Geometry: final body of the model. Coordinates: model frame, mm. A direction names the side the tool comes from. Give positions to 0.01 mm unless a question says otherwise; leave off trailing zeros. Loops run counter-clockwise (first coordinate to the right, second up) from the corner with the lowest first, then second, coordinate; pieces in that order, holes last.
1. First-contact query: P1, Ø16, axis at x = 4, y = 30.5, coming from the -Z side; P2, Ø1.9, axis at x = -3, z = 108, coming from the -Y side; P3, Ø5, axis at x = -7.75, z = 116, coming from the +Y side. Flat tips, straight axial feed; report the tip coordinate or a pass-through.
2. Material intervals for line 1 along Y through (x, z) = (-1, 118); line 2 along X through (y, z) = (-23, 100); line 3 along X through (y, z) = (23, 93), sorted ascending.
3. Access query for faces 3 (the face through (11, 28, 126)), 4 (the face through (11.131, -55.528, 114.997)), 5 (the face through (0.808, -23.965, 90.978)), 6 (the face through (13, 0, 108)), 7 (the face through (15, 35, 108)). Directions: +Z, -Z, +X, -X, +Y, -Y. A direction counts if a zero-diameter tool reaches every point of the face in a straight line with its end or side. Return the directions, or none.
4. Section C-C, the plane y = -47. Output: boundary loops of the cut face in (x, z), then the cut area to 3 significant figures.
5. Draft query along Z for faces 1 (the face through (7.845, -23.528, 94.124)), 2 (the face through (-12, -55, 108)). Return one class per face: +Z half, -Z half, draft (parallel to the pull), parting line (faces both ways), or undercut.
6. Section B-B, the plane z = 108. State how many separate pieces and enclosed holes the cut face has, then the cut area to 3 significant figures.
7. Section A-A, the plane y = -31.5. Output: boundary loops of the cut face in (x, z).
from build123d import *

# Parameters (mm, degrees)
SKETCH_W               = 51
SKETCH_H               = 40
PAD_DEPTH              = 6
SKETCH002_W            = 4
SKETCH002_H            = 40
PAD001_DEPTH           = 25
PAD009_DEPTH           = 20
SKETCH031_W            = 5.9
SKETCH031_H            = 12.9
POCKET009_DEPTH        = 40
PAD010_DEPTH           = 12
SKETCH032_R            = 1.6
SKETCH032_R_2          = 1.025
POCKET010_DEPTH        = 5
SKETCH033_R            = 1.6
POCKET011_DEPTH        = 5
POCKET012_DEPTH        = 5
SKETCH042_R            = 1.6
POCKET019_DEPTH        = 5
SKETCH043_R            = 1.025
POCKET020_DEPTH        = 5
LINEARPATTERN004_COUNT = 2
LINEARPATTERN004_PITCH = 32
SKETCH044_W            = 4
SKETCH044_H            = 32
PAD015_DEPTH           = 27
SKETCH045_R            = 6
SKETCH045_R_2          = 2.1
POCKET021_DEPTH        = 5
FILLET001_R            = 1


with BuildPart() as part:
    # Sketch → Pad (new body)
    with BuildSketch(Plane.YZ):
        Rectangle(SKETCH_W, SKETCH_H)
    extrude(amount=PAD_DEPTH)

    # Sketch002 (on Face5 of Pad) → Pad001 (join)
    with BuildSketch(Plane(origin=(0, 0, 0), x_dir=(0, 1, 0), z_dir=(-1, 0, 0))):
        with Locations((23.5, 0)):
            Rectangle(SKETCH002_W, SKETCH002_H)
        with Locations((-23.5, 0)):
            Rectangle(SKETCH002_W, SKETCH002_H)
    extrude(amount=PAD001_DEPTH)

    # Sketch030 (on Face9 of Pad001) → Pad009 (join)
    with BuildSketch(Plane.ZX.offset(25.5)):
        Polygon((-16, -25), (-20, -25), (-20, 6), (20, 6), (20, -25), (16, -25), (16, 2), (-16, 2), align=None)
    pad009 = extrude(amount=PAD009_DEPTH)

    # Sketch031 (on Face12 of Pad009) → Pocket009 (cut)
    with BuildSketch(Plane.YX.offset(20)):
        Polygon((27.5, -25), (45.5, 0), (45.5, -25), align=None)
        with Locations((28.45, -8.45)):
            Rectangle(SKETCH031_W, SKETCH031_H)
    extrude(amount=-POCKET009_DEPTH, mode=Mode.SUBTRACT)

    # Mirrored: Pad009 across XZ
    add(pad009.mirror(Plane.XZ))

    # Mirrored Face21 → Pad010 (add)
    with BuildSketch(Plane(origin=(-4.904255, -45.5, 0), x_dir=(-1, 0, 0), z_dir=(0, -1, 0))):
        Polygon((20.095745, 16), (20.095745, 20), (-10.904255, 20), (-10.904255, -20), (20.095745, -20), (20.095745, -16), (-6.904255, -16), (-6.904255, 16), align=None)
    extrude(amount=PAD010_DEPTH)

    # Sketch032 (on Face19 of Pad010) → Pocket010 (cut)
    with BuildSketch(Plane(origin=(0, -25.5, 0), x_dir=(0, 0, -1), z_dir=(0, -1, 0))):
        with Locations((-8, -5.75)):
            Circle(SKETCH032_R)
        with Locations((8, -5.75)):
            Circle(SKETCH032_R)
        with Locations((8, -20.75)):
            Circle(SKETCH032_R)
        with Locations((-8, -20.75)):
            Circle(SKETCH032_R)
        with Locations((-14.9, -5.2)):
            Circle(SKETCH032_R_2)
        with Locations((-14.9, -11.7)):
            Circle(SKETCH032_R_2)
        with Locations((14.9, -5.2)):
            Circle(SKETCH032_R_2)
        with Locations((14.9, -11.7)):
            Circle(SKETCH032_R_2)
        with Locations((0, -16)):
            Circle(SKETCH032_R)
        with Locations((0, -22)):
            Circle(SKETCH032_R)
    pocket010 = extrude(amount=-POCKET010_DEPTH, mode=Mode.SUBTRACT)

    # Mirrored001: Pocket010 across XZ
    add(pocket010.mirror(Plane.XZ), mode=Mode.SUBTRACT)

    # Sketch033 (on Face30 of Mirrored001) → Pocket011 (cut)
    with BuildSketch(Plane.YZ.offset(6)):
        with Locations((-27, 8.5)):
            Circle(SKETCH033_R)
        with Locations((28, 8.5)):
            Circle(SKETCH033_R)
        with Locations((28, -8.5)):
            Circle(SKETCH033_R)
        with Locations((-27, -8.5)):
            Circle(SKETCH033_R)
    extrude(amount=-POCKET011_DEPTH, mode=Mode.SUBTRACT)

    # Sketch034 (on Face48 of Pocket011) → Pocket012 (cut)
    with BuildSketch(Plane(origin=(2, 0, 0), x_dir=(0, 1, 0), z_dir=(-1, 0, 0))):
        Polygon((-27.5, -5.42), (-30.167358, -6.96), (-30.167358, -10.04), (-27.5, -11.58), (-24.832642, -10.04), (-24.832642, -6.96), align=None)
    extrude(amount=POCKET012_DEPTH, mode=Mode.SUBTRACT)

    # Sketch042 (on Face13 of Pocket012) → Pocket019 (cut)
    with BuildSketch(Plane.YX.offset(20)):
        with Locations((-31.5, -12.5)):
            Circle(SKETCH042_R)
        with Locations((-51.5, -12.5)):
            Circle(SKETCH042_R)
    pocket019 = extrude(amount=-POCKET019_DEPTH, mode=Mode.SUBTRACT)

    # Mirrored005: Pocket019 across XY
    add(pocket019.mirror(Plane.XY), mode=Mode.SUBTRACT)

    # Sketch043 (on Face27 of Mirrored005) → Pocket020 (cut)
    with BuildSketch(Plane.ZX.offset(-21.5)):
        with Locations((-18, -12.5)):
            Circle(SKETCH043_R)
        with Locations((-18, -4.5)):
            Circle(SKETCH043_R)
    pocket020 = extrude(amount=-POCKET020_DEPTH, mode=Mode.SUBTRACT)

    # LinearPattern004: Pocket020 ×2
    with Locations(*[(0, -i * LINEARPATTERN004_PITCH, 0) for i in range(1, LINEARPATTERN004_COUNT)]):
        add(pocket020, mode=Mode.SUBTRACT)

    # Sketch044 (on Face54 of LinearPattern004) → Pad015 (join)
    with BuildSketch(Plane(origin=(2, 0, 0), x_dir=(0, 1, 0), z_dir=(-1, 0, 0))):
        with Locations((-55.5, 0)):
            Rectangle(SKETCH044_W, SKETCH044_H)
    extrude(amount=PAD015_DEPTH)

    # Sketch045 (on Face64 of Pad015) → Pocket021 (cut)
    with BuildSketch(Plane(origin=(0, -57.5, 0), x_dir=(0, 0, -1), z_dir=(0, -1, 0))):
        with Locations((0, -11.5)):
            Circle(SKETCH045_R)
        with Locations((-9, -2.5)):
            Circle(SKETCH045_R_2)
        with Locations((9, -2.5)):
            Circle(SKETCH045_R_2)
        with Locations((9, -20.5)):
            Circle(SKETCH045_R_2)
        with Locations((-9, -20.5)):
            Circle(SKETCH045_R_2)
    extrude(amount=-POCKET021_DEPTH, mode=Mode.SUBTRACT)

    # Fillet001
    fillet001_edges = [part.edges().sort_by_distance(p)[0] for p in [
        (-25, -57.5, 0),
        (6, -6, -20),
        (-9.5, -57.5, 20),
        (6, -6, 20),
        (-25, -39.5, 20),
        (-25, -39.5, -20),
        (-25, -21.5, 0),
        (-25, 27.5, -18),
        (-12.5, 36.5, -20),
        (-25, 25.5, 0),
        (-25, 27.5, 18),
        (3, 45.5, -20),
        (3, 45.5, 20),
        (-12.5, 36.5, 20),
        (0, 0, 20),
        (0, 0, -20),
        (6, -57.5, 0),
        (-25, 24.5, 20),
        (-25, 24.5, -20),
        (-25, 21.5, 0),
        (2, 45.5, 0),
        (-12.5, 36.5, 16),
        (-12.5, 36.5, -16),
        (0, 45.5, -18),
        (0, 45.5, 18),
        (1, 45.5, 16),
        (6, 45.5, 0),
    ]]
    fillet(fillet001_edges, radius=FILLET001_R)


with BuildPart() as part_1:
    # Body placement: moved
    add(part.part.moved(Location((13, 0, 108))))


solid = part_1.part
Answers below:
1. P1: stops at z = 88
1. P2: passes through
1. P3: stops at y = 25.5
2. line 1: y = -57.5 to -53.5, -25.5 to -21.5, 21.5 to 25.5
2. line 2: x = -12 to -9.35, -6.15 to 5.65, 8.85 to 19
2. line 3: x = -12 to 0.28, 2.32 to 6.78, 8.82 to 19
3. face 3: +Z, -Z
3. face 4: -Y
3. face 5: none
3. face 6: +Z, -Z, -X
3. face 7: -X, +Y
4. outline: (-12, 89) arc R1 ccw to (-11, 88) - (18, 88) arc R1 ccw to (19, 89) - (19, 127) arc R1 ccw to (18, 128) - (-11, 128) arc R1 ccw to (-12, 127) - (-12, 124) - (15, 124) - (15, 92) - (-12, 92) - close
4. area: 375 mm2
5. face 1: undercut
5. face 2: draft
6. separate pieces: 6
6. enclosed holes: 0
6. area: 721 mm2
7. outline: (-12, 89) arc R1 ccw to (-11, 88) - (-1.1, 88) - (-1.1, 92) - (-12, 92) - close; (-12, 124) - (-1.1, 124) - (-1.1, 128) - (-11, 128) arc R1 ccw to (-12, 127) - close; (2.1, 88) - (18, 88) arc R1 ccw to (19, 89) - (19, 127) arc R1 ccw to (18, 128) - (2.1, 128) - (2.1, 124) - (15, 124) - (15, 92) - (2.1, 92) - close
